Can you work these out from the model? Positions are in its coordinate system, mm. A direction names the side the tool comes from. Round coordinates to 2 decimals unless told otherwise and drop trailing zeros. Write each loop counter-clockwise with the first axis right and the second up, starting at its lowest first coordinate (ties: lowest second). Pieces come first, ordered by that corner, then holes. Notation, with made-up numbers: M 52.5,45.5 L 56.5,45.5 A8 cw 56.5,59.5 Z; hole C 30,12.25 d5. An arc over 180 degrees is marked long. Use one line per item in the form item = value. Start each with the question number.
```python
from build123d import *

# Parameters (mm, degrees)
SKETCH1_R           = 15
BOSS_EXTRUDE1_DEPTH = 620
SKETCH2_R           = 13.5
CUT_EXTRUDE1_DEPTH  = 621.362797079
SKETCH4_R           = 16.267367871
SKETCH4_R_2         = 14.447843326
CUT_EXTRUDE2_DEPTH  = 30
SKETCH5_R           = 16.193324777
SKETCH5_R_2         = 14.662495413
CUT_EXTRUDE3_DEPTH  = 21


with BuildPart() as part:
    # Sketch1 → Boss-Extrude1 (new body)
    with BuildSketch(Plane.XY):
        Circle(SKETCH1_R)
    extrude(amount=BOSS_EXTRUDE1_DEPTH)

    # Sketch2 → Cut-Extrude1 (cut, through all)
    with BuildSketch(Plane(origin=(0, 0, 0), x_dir=(-1, 0, 0), z_dir=(0, 0, -1))):
        Circle(SKETCH2_R)
    extrude(amount=-CUT_EXTRUDE1_DEPTH, mode=Mode.SUBTRACT)

    # Sketch4 → Cut-Extrude2 (cut)
    with BuildSketch(Plane.XY.offset(480)):
        Circle(SKETCH4_R)
        Circle(SKETCH4_R_2, mode=Mode.SUBTRACT)
    cut_extrude2 = extrude(amount=CUT_EXTRUDE2_DEPTH, mode=Mode.SUBTRACT)

    # Mirror1: Cut-Extrude2 across plane
    add(cut_extrude2.mirror(Plane.XY.offset(310)), mode=Mode.SUBTRACT)

    # Sketch5 → Cut-Extrude3 (cut)
    with BuildSketch(Plane.XY.offset(620)):
        Circle(SKETCH5_R)
        Circle(SKETCH5_R_2, mode=Mode.SUBTRACT)
    cut_extrude3 = extrude(amount=-CUT_EXTRUDE3_DEPTH, mode=Mode.SUBTRACT)

    # Mirror2: Cut-Extrude3 across plane
    add(cut_extrude3.mirror(Plane.XY.offset(310)), mode=Mode.SUBTRACT)


solid = part.part
```
1. If we mould it in two halves opening along Z, with no side actions, what happens to faces 3 (the face through (2.93, -13.18, 305.66)), 4 (the face through (6.6, -13.3, 599)), 5 (the face through (6.6, -13.3, 21)), 6 (the face through (-3.132, -14.104, 494.79))? For each: pulls with the +Z half, pulls with the -Z half, needs draft (parallel to the pull), parting line crosses it, or undercut.
2. Will these pins go through, and if not, where does the flat tip stop? pin 1 (10 mm diameter, centred on x = -11, z = 196, fed in from +Y); pin 2 (5 mm diameter, centred on y = -2.5, z = 367, fed in from +X); pin 3 (10 mm diameter, centred on x = 7.5, z = 491, fed in from -Y); pin 4 (15 mm diameter, centred on x = -4, y = -4, fed in from -Z).
3. Please list where these lines run through material, in increasing order: line 1 along Y through (x, z) = (0, 165); line 2 along Y through (x, z) = (0, 129.5); line 3 along X through (y, z) = (-4.75, 193.5).
4. Which directions (+Z, -Z, +X, -X, +Y, -Y) give clear straight access to the entire face, cutting with the end or side of a thin tool? Please do faces 1 (the face through (-3.132, -14.104, 125.21)), 2 (the face through (13, -4.3, 620)).
5. If we section it at C-C (z = 349): List the corners of the cut face in (x, y) for me, and give its area (3 significant figures).
Model answer:
q1.face_3 = needs draft
q1.face_4 = pulls with the +Z half
q1.face_5 = pulls with the -Z half
q1.face_6 = undercut
q2.pin_1 = 13.75
q2.pin_2 = 15
q2.pin_3 = -14.23
q2.pin_4 = through
q3.line_1 = -15 to -13.5, 13.5 to 15
q3.line_2 = -14.45 to -13.5, 13.5 to 14.45
q3.line_3 = -14.23 to -12.64, 12.64 to 14.23
q4.face_1 = none
q4.face_2 = +Z, +X, -X, +Y, -Y
q5.outline = C 0,0 d30; hole C 0,0 d27
q5.area = 134 mm2
